from build123d import *

# Parameters (mm, degrees)
SKETCH2_R           = 6.5
BOSS_EXTRUDE1_DEPTH = 2
BOSS_EXTRUDE2_DEPTH = 90.25
BOSS_EXTRUDE3_START = 90.25
SKETCH2_4_R         = 6.5
BOSS_EXTRUDE3_DEPTH = 3
BOSS_EXTRUDE4_DEPTH = 20
BOSS_EXTRUDE5_START = 5
BOSS_EXTRUDE5_DEPTH = 15
SKETCH4_R           = 18
SKETCH4_R_2         = 12
BOSS_EXTRUDE6_DEPTH = 3


with BuildPart() as part:
    # Sketch2 → Boss-Extrude1 (new body)
    with BuildSketch(Plane(origin=(0, 0, 0), x_dir=(1, 0, 0), z_dir=(0, 1, 0))):
        with BuildLine():
            Line((-43.540750747, 45.85713332), (-27.367167941, 27.4))
            Line((-27.367167941, 27.4), (-27.367167941, -25.4))
            Line((-27.367167941, -25.4), (27.4, -25.4))
            Line((27.4, -25.4), (27.4, 38.429357381))
            Line((27.4, 38.429357381), (-15.776081894, 38.429357381))
            Line((-15.776081894, 38.429357381), (-32.466678415, 55.970011272))
            ThreePointArc((-32.466678415, 55.970011272), (-42.957502529, 56.338200806), (-43.540750747, 45.85713332))
        make_face()
        with Locations(Location((-37.9, 50.8, 0), (0, 0, 270))):
            Circle(SKETCH2_R, mode=Mode.SUBTRACT)
    extrude(amount=BOSS_EXTRUDE1_DEPTH)

    # Sketch2<3> → Boss-Extrude2 (add)
    with BuildSketch(Plane(origin=(0, 0, 0), x_dir=(1, 0, 0), z_dir=(0, 1, 0))):
        Polygon((-24.867167941, -23.4), (-27.367167941, -25.4), (27.4, -25.4), (27.4, 38.429357381), (25.4, 38.429357381), (25.4, -23.4), align=None)
    extrude(amount=BOSS_EXTRUDE2_DEPTH)

    # Sketch2<4> → Boss-Extrude3 (add)
    with BuildSketch(Plane(origin=(0, 0, 0), x_dir=(1, 0, 0), z_dir=(0, 1, 0)).offset(BOSS_EXTRUDE3_START)):
        with BuildLine():
            Line((-43.540750747, 45.85713332), (-27.367167941, 27.4))
            Line((-27.367167941, 27.4), (-27.367167941, -25.4))
            Line((-27.367167941, -25.4), (27.4, -25.4))
            Line((27.4, -25.4), (27.4, 38.429357381))
            Line((27.4, 38.429357381), (-15.776081894, 38.429357381))
            Line((-15.776081894, 38.429357381), (-32.466678415, 55.970011272))
            ThreePointArc((-32.466678415, 55.970011272), (-42.957502529, 56.338200806), (-43.540750747, 45.85713332))
        make_face()
        with Locations(Location((-37.9, 50.8, 0), (0, 0, 270))):
            Circle(SKETCH2_4_R, mode=Mode.SUBTRACT)
    extrude(amount=BOSS_EXTRUDE3_DEPTH)

    # Sketch3 → Boss-Extrude4 (add)
    with BuildSketch(Plane(origin=(27.4, 0, 0), x_dir=(0, 0, -1), z_dir=(1, 0, 0))):
        with BuildLine():
            ThreePointArc((-18.4, 41.650062814), (-22.9, 46.625), (-18.4, 51.599937186))
            Line((-18.4, 51.599937186), (-18.4, 54.108314774))
            ThreePointArc((-18.4, 54.108314774), (-25.4, 46.625), (-18.4, 39.141685226))
            Line((-18.4, 39.141685226), (-18.4, 41.650062814))
        make_face()
        with BuildLine():
            Line((-17.4, 54.108314774), (-17.4, 51.599937186))
            ThreePointArc((-17.4, 51.599937186), (-12.9, 46.625), (-17.4, 41.650062814))
            Line((-17.4, 41.650062814), (-17.4, 39.141685226))
            ThreePointArc((-17.4, 39.141685226), (-10.4, 46.625), (-17.4, 54.108314774))
        make_face()
    extrude(amount=BOSS_EXTRUDE4_DEPTH)

    # Sketch3<3> → Boss-Extrude5 (add)
    with BuildSketch(Plane(origin=(27.4, 0, 0), x_dir=(0, 0, -1), z_dir=(1, 0, 0)).offset(BOSS_EXTRUDE5_START)):
        with BuildLine():
            ThreePointArc((-25.4, 46.625), (-23.377225575, 51.748475383), (-18.4, 54.108314774))
            Line((-18.4, 54.108314774), (-18.4, 58.125))
            Line((-18.4, 58.125), (-25.4, 58.125))
            Line((-25.4, 58.125), (-25.4, 46.625))
        make_face()
        with BuildLine():
            Line((-17.4, 58.125), (-17.4, 54.108314774))
            ThreePointArc((-17.4, 54.108314774), (-12.422774425, 51.748475383), (-10.4, 46.625))
            Line((-10.4, 46.625), (-10.4, 58.125))
            Line((-10.4, 58.125), (-17.4, 58.125))
        make_face()
        with BuildLine():
            ThreePointArc((-18.4, 39.141685226), (-23.377225575, 41.501524617), (-25.4, 46.625))
            Line((-25.4, 46.625), (-25.4, 35.125))
            Line((-25.4, 35.125), (-18.4, 35.125))
            Line((-18.4, 35.125), (-18.4, 39.141685226))
        make_face()
        with BuildLine():
            Line((-10.4, 35.125), (-10.4, 46.625))
            ThreePointArc((-10.4, 46.625), (-12.422774425, 41.501524617), (-17.4, 39.141685226))
            Line((-17.4, 39.141685226), (-17.4, 35.125))
            Line((-17.4, 35.125), (-10.4, 35.125))
        make_face()
    extrude(amount=BOSS_EXTRUDE5_DEPTH)

    # Sketch4 → Boss-Extrude6 (add)
    # profile 1 of 3: a face of its own
    with BuildSketch(Plane.XZ):
        with Locations((46.65, -28.429357381)):
            Circle(SKETCH4_R)
        with Locations(Location((46.65, -28.429357381, 0), (0, 0, 270))):
            Circle(SKETCH4_R_2, mode=Mode.SUBTRACT)
    # profile 2 of 3: a face of its own
    with BuildSketch(Plane.XZ):
        with BuildLine():
            Line((27.4, -17.315364699), (27.4, -38.429357381))
            Line((27.4, -38.429357381), (38.026563161, -44.229241465))
            ThreePointArc((38.026563161, -44.229241465), (30.850115916, -19.805920542), (55.273436839, -12.629473297))
            Line((55.273436839, -12.629473297), (45.117240383, -7.086311195))
            Line((45.117240383, -7.086311195), (27.4, -17.315364699))
        make_face()
    # profile 3 of 3: a face of its own
    with BuildSketch(Plane.XZ):
        Polygon((27.4, 2.583601736), (27.4, -17.315364699), (45.117240383, -7.086311195), align=None)
    extrude(amount=-BOSS_EXTRUDE6_DEPTH)


solid = part.part
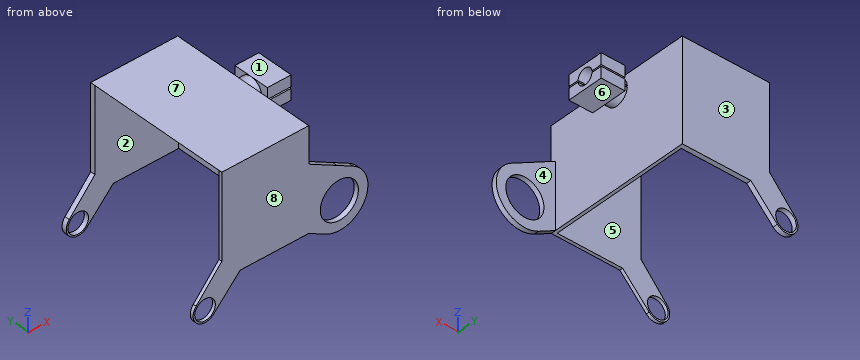
Here's how the part is built. I have some questions about the finished solid (model axes, mm). Face numbers are marked on the shaded views. A direction names the side the tool comes from. Coordinates: 2 decimals unless noted, no trailing zeros. Write each loop counter-clockwise with the first axis right and the second up, starting at its lowest first coordinate (ties: lowest second). Pieces come first, ordered by that corner, then holes.
1) If we section it at A-A (z = 9): List the corners of the cut face in (x, y) for me.
Filled in:
outline: (-27.37, 0) - (27.4, 0) - (27.4, 93.25) - (-27.37, 93.25) - (-27.37, 90.25) - (25.4, 90.25) - (25.4, 2) - (-27.37, 2) - close
2) If we section it at B-B (x = 36): List the corners of the cut face in (y, z) for me (3 decimals).
Filled in:
outline: (0, -43.123) - (3, -43.123) - (3, -33.959) - (0, -33.959) - close; (0, -22.9) - (3, -22.9) - (3, -2.11) - (0, -2.11) - close; (35.125, 10.4) - (58.125, 10.4) - (58.125, 17.4) - (51.6, 17.4) arc R5 cw to (41.65, 17.4) - (35.125, 17.4) - close; (35.125, 18.4) - (41.65, 18.4) arc R5 cw to (51.6, 18.4) - (58.125, 18.4) - (58.125, 25.4) - (35.125, 25.4) - close
3) If we section it at C-C (x = 4): List the corners of the cut face in (y, z) for me.
Filled in:
outline: (0, -38.43) - (2, -38.43) - (2, 23.4) - (90.25, 23.4) - (90.25, -38.43) - (93.25, -38.43) - (93.25, 25.4) - (0, 25.4) - close
4) If we section it at D-D (z = -20.5): List the corners of the cut face in (x, y) for me, plus the area to 3 significant figures.
Filled in:
outline: (-27.37, 0) - (37.64, 0) - (37.64, 3) - (27.4, 3) - (27.4, 93.25) - (-27.37, 93.25) - (-27.37, 90.25) - (25.4, 90.25) - (25.4, 2) - (-27.37, 2) - close; (55.66, 0) - (62.81, 0) - (62.81, 3) - (55.66, 3) - close
area: 503 mm2
5) Thinking about a two-plate mould opening in Y: for the marked faces 1, 2 and 3, which applies, +Y half, -Y half, draft (parallel to the pull), parting line (faces both ways), or undercut?
Filled in:
face 1: draft
face 2: undercut
face 3: +Y half
6) I'm going to push flat-ended pins straight in: pin 1 (7.5 mm diameter, centred on y = 49, z = 15.5, fed in from +X); pin 2 (10 mm diameter, centred on y = 69, z = 10, fed in from +X); pin 3 (18.5 mm diameter, centred on y = 29.5, z = -5.5, fed in from -X); pin 4 (6 mm diameter, centred on y = 70, z = -44, fed in from -X). Where does each tip first touch, or does it pass through?
Filled in:
pin 1: stops at x = 47.4
pin 2: stops at x = 27.4
pin 3: stops at x = 25.4
pin 4: passes through
7) If I drill on line 1 (Y direction, x = 1.5, z = -4); line 2 (Z direction, x = -22, y = 77); line 3 (X direction, y = 91, z = -50), over which ranges is the centre line in solid material (lowest first)?
Filled in:
line 1: y = 0 to 2, 90.25 to 93.25
line 2: z = 23.4 to 25.4
line 3: x = -45.36 to -44.35, -31.45 to -26.79
8) Which directions (+Z, -Z, +X, -X, +Y, -Y) give clear straight access to the entire face, cutting with the end or side of a thin tool? Please do the marked faces 4, 5, 6, 7 and 8.
Filled in:
face 4: +Z, -Z, +X, +Y
face 5: -Z, -X
face 6: -Z, +X, +Y, -Y
face 7: +Z, +X, -X, +Y, -Y
face 8: +Z, -Z, +X, -X, -Y
